CAD build for the part. Positions are in the model's coordinates, mm. Face numbers are marked on the shaded views. A direction names the side the tool comes from. Round coordinates to 2 decimals unless told otherwise and drop trailing zeros. Loops run counter-clockwise (first coordinate to the right, second up) from the corner with the lowest first, then second, coordinate; pieces in that order, holes last. Notation, with made-up numbers: M 53.25,2 L 62.25,2 A11 cw 62.25,11 Z; hole C 61.5,-7 d2. An arc over 180 degrees is marked long. Use a Markdown table: item, result. Add a question column.
(1) Which spindle directions (+Z, -Z, +X, -X, +Y, -Y) get a long thin tool onto all of the face, cutting with end or side? Do the marked faces 5 and 6. Say none if no direction does.
(2) Band-saw the part on B-B, the plane y = -22.5. Write the cut outline in (x, z).
(3) Band-saw the part on C-C, the plane x = 0. Write the cut outline in (y, z).
(4) Band-saw the part on A-A, the plane z = -5.5. Write the cut outline in (x, y).
(5) Two-plate mould, pull along X, no slides. Class the marked faces 1, 2, 3 and 4: released by +X, released by -X, zero draft, split by the parting line, or undercut.
(6) Flat gauge pin, fed straight in: P1, Ø5.5, axis at x = 4.5, y = 4.5, coming from the +Z side. Where does the tip first touch, or does it go through?
(7) Wall check: L1, parallel to X at y = 1, z = -2; L2, parallel to Z at x = -13.5, y = -5; L3, parallel to Z at x = -28, y = 1. Give the ranges that are in metal, low to high.
from build123d import *

# Parameters (mm, degrees)
F1_DEPTH = 30
F3_DEPTH = 100
F5_DEPTH = 2
F7_DEPTH = 2
F9_DEPTH = 2


with BuildPart() as f1:
    # F0 (on Front) → F1 (new body, symmetric)
    with BuildSketch(Plane.XZ):
        Polygon((-54, 89.197368), (-54, -34.802632), (54, -34.802632), (54, 89.197368), (44, 89.197368), (44, -18.802632), (-44, -18.802632), (-44, 89.197368), align=None)
    extrude(amount=F1_DEPTH, both=True)

    # F2 (on Right) → F3 (cut, symmetric)
    with BuildSketch(Plane.YZ):
        with BuildLine():
            Line((-11.05, 89.197368), (-11.05, 86.197368))
            ThreePointArc((-11.05, 86.197368), (0, 75.147368), (11.05, 86.197368))
            Line((11.05, 86.197368), (11.05, 89.197368))
            Line((11.05, 89.197368), (-11.05, 89.197368))
        make_face()
    extrude(amount=F3_DEPTH, both=True, mode=Mode.SUBTRACT)

    # F4 (on face) → F5 (cut)
    with BuildSketch(Plane.XY.offset(-18.802632)):
        with BuildLine():
            ThreePointArc((-35.216444, 15), (-36.630658, 14.414214), (-37.216444, 13))
            Line((-37.216444, 13), (-37.216444, -13))
            ThreePointArc((-37.216444, -13), (-36.630658, -14.414214), (-35.216444, -15))
            ThreePointArc((-35.216444, -15), (-33.80223, -14.414214), (-33.216444, -13))
            Line((-33.216444, -13), (-33.216444, 2.259175))
            ThreePointArc((-33.216444, 2.259175), (-32.806176, 2.751057), (-32.248652, 2.435726))
            Line((-32.248652, 2.435726), (-29.619821, -4.529654))
            ThreePointArc((-29.619821, -4.529654), (-28.216444, -5.5), (-26.813067, -4.529654))
            Line((-26.813067, -4.529654), (-24.184236, 2.435726))
            ThreePointArc((-24.184236, 2.435726), (-23.626711, 2.751057), (-23.216444, 2.259175))
            Line((-23.216444, 2.259175), (-23.216444, -13))
            ThreePointArc((-23.216444, -13), (-22.630658, -14.414214), (-21.216444, -15))
            ThreePointArc((-21.216444, -15), (-19.80223, -14.414214), (-19.216444, -13))
            Line((-19.216444, -13), (-19.216444, 13))
            ThreePointArc((-19.216444, 13), (-19.80223, 14.414214), (-21.216444, 15))
            Line((-21.216444, 15), (-21.904706, 15))
            ThreePointArc((-21.904706, 15), (-23.001574, 14.672388), (-23.739094, 13.796882))
            Line((-23.739094, 13.796882), (-27.29925, 5.601559))
            ThreePointArc((-27.29925, 5.601559), (-28.216444, 5), (-29.133638, 5.601559))
            Line((-29.133638, 5.601559), (-32.693794, 13.796882))
            ThreePointArc((-32.693794, 13.796882), (-33.431314, 14.672388), (-34.528182, 15))
            Line((-34.528182, 15), (-35.216444, 15))
        make_face()
    extrude(amount=-F5_DEPTH, mode=Mode.SUBTRACT)

    # F6 (on face) → F7 (cut)
    with BuildSketch(Plane.XY.offset(-18.802632)):
        with BuildLine():
            Line((-8.361575, 15), (-8.361575, -15))
            ThreePointArc((-8.361575, -15), (9.638425, 0), (-8.361575, 15))
        make_face()
        with BuildLine():
            Line((-4.961575, -11), (-4.961575, 11))
            ThreePointArc((-4.961575, 11), (6.038425, 0), (-4.961575, -11))
        make_face(mode=Mode.SUBTRACT)
    extrude(amount=-F7_DEPTH, mode=Mode.SUBTRACT)

    # F8 (on face) → F9 (cut)
    with BuildSketch(Plane.XY.offset(-18.802632)):
        Polygon((19.817374, 15), (19.817374, -15), (35.817374, -15), (35.817374, -10), (24.817374, -10), (24.817374, -2.5), (34.817374, -2.5), (34.817374, 2.5), (24.817374, 2.5), (24.817374, 10), (35.817374, 10), (35.817374, 15), align=None)
    extrude(amount=-F9_DEPTH, mode=Mode.SUBTRACT)


solid = f1.part
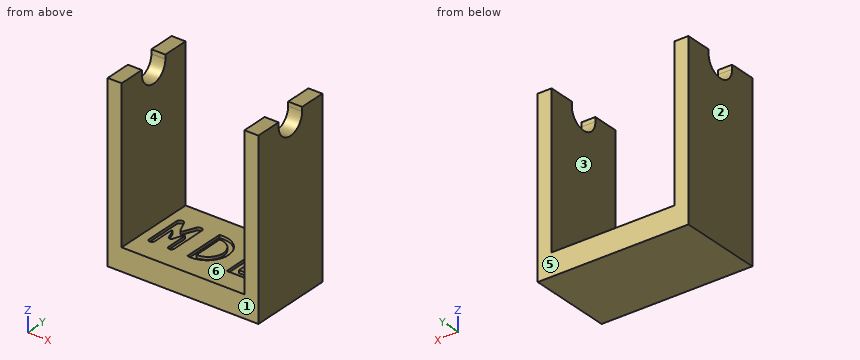
Return value:
| question | item | result |
|---|---|---|
| 1 | face 5 | +Z, -Z, +X, -X, +Y |
| 1 | face 6 | +Z, +Y, -Y |
| 2 | outline | M -54,-34.8 L 54,-34.8 L 54,89.2 L 44,89.2 L 44,-18.8 L -44,-18.8 L -44,89.2 L -54,89.2 Z |
| 3 | outline | M -30,-34.8 L 30,-34.8 L 30,-18.8 L 14.18,-18.8 L 14.18,-20.8 L 9.82,-20.8 L 9.82,-18.8 L -9.82,-18.8 L -9.82,-20.8 L -14.18,-20.8 L -14.18,-18.8 L -30,-18.8 Z |
| 4 | outline | M -54,-30 L -44,-30 L -44,30 L -54,30 Z; M 44,-30 L 54,-30 L 54,30 L 44,30 Z |
| 5 | face 1 | zero draft |
| 5 | face 2 | released by -X |
| 5 | face 3 | undercut |
| 5 | face 4 | undercut |
| 6 | P1 | z = -18.8 |
| 7 | L1 | -54 to -44, 44 to 54 |
| 7 | L2 | -34.8 to -18.8 |
| 7 | L3 | -34.8 to -20.8 |
